```python
from build123d import *

# Parameters (mm, degrees)
BOSS_EXTRUDE1_DEPTH = 1
SKETCH2_R           = 1.6
SKETCH2_W           = 161.4
SKETCH2_H           = 58.6
CUT_EXTRUDE1_DEPTH  = 211.355512163


with BuildPart() as part:
    # Sketch1 → Boss-Extrude1 (new body)
    with BuildSketch(Plane(origin=(0, 0, 0), x_dir=(1, 0, 0), z_dir=(0, 1, 0))):
        with BuildLine():
            Line((92, 0), (-92, 0))
            add(Edge.make_bspline(
                [(-92, 0), (-99, 0), (-100, 8)],
                knots=[0, 0, 0, 1, 1, 1], degree=2))
            add(Edge.make_bspline(
                [(-100, 8), (-109.749547472, 87.403692131), (-94, 164)],
                knots=[0, 0, 0, 1, 1, 1], degree=2))
            add(Edge.make_bspline(
                [(-94, 164), (-90, 183), (-80, 183)],
                knots=[0, 0, 0, 1, 1, 1], degree=2))
            Line((-80, 183), (80, 183))
            add(Edge.make_bspline(
                [(94, 164), (90, 183), (80, 183)],
                knots=[0, 0, 0, 1, 1, 1], degree=2))
            add(Edge.make_bspline(
                [(100, 8), (109.749547472, 87.403692131), (94, 164)],
                knots=[0, 0, 0, 1, 1, 1], degree=2))
            add(Edge.make_bspline(
                [(92, 0), (99, 0), (100, 8)],
                knots=[0, 0, 0, 1, 1, 1], degree=2))
        make_face()
    extrude(amount=BOSS_EXTRUDE1_DEPTH)

    # Sketch2 → Cut-Extrude1 (cut, through all)
    with BuildSketch(Plane(origin=(0, 1, 0), x_dir=(1, 0, 0), z_dir=(0, 1, 0))):
        with Locations(Location((-88, 3.5, 0), (0, 0, 270))):
            Circle(SKETCH2_R)
        with Locations(Location((88, 3.5, 0), (0, 0, 90))):
            Circle(SKETCH2_R)
        with Locations(Location((-80, 175, 0), (0, 0, 270))):
            Circle(SKETCH2_R)
        with Locations(Location((80, 175, 0), (0, 0, 90))):
            Circle(SKETCH2_R)
        with Locations(Location((-88, 68.5, 0), (0, 0, 270))):
            Circle(SKETCH2_R)
        with Locations(Location((88, 68.5, 0), (0, 0, 270))):
            Circle(SKETCH2_R)
        with Locations((-1.3, 43.6)):
            Rectangle(SKETCH2_W, SKETCH2_H)
    extrude(amount=-CUT_EXTRUDE1_DEPTH, mode=Mode.SUBTRACT)


solid = part.part
```
Work out the finished part from the listing and answer in its coordinate system (mm). Round coordinates to 2 decimals unless told otherwise and drop trailing zeros. Loops run counter-clockwise (first coordinate to the right, second up) from the corner with the lowest first, then second, coordinate; pieces in that order, holes last. Notation, with made-up numbers: M -27,70.5 L 13,70.5 A11 cw 13,87.5 Z; hole C -8.75,-10 d2. An arc over 180 degrees is marked long. One line per question, with ' | ' between items.
Q1. Find section A-A, the plane x = 11.5. Give the vertices of the cut face in (y, z).
Conclusion:
outline: M 0,-183 L 1,-183 L 1,-72.9 L 0,-72.9 Z; M 0,-14.3 L 1,-14.3 L 1,0 L 0,0 Z
Q2. Find section B-B, the plane y = 0.75. State how many separate pieces and enclosed holes the cut face has, then the cut area to 3 significant figures.
Conclusion:
separate pieces: 1 | enclosed holes: 7 | area: 27,100 mm2
Q3. This flat-tipped pin is pushed along its axis until it touches: pin 1 Ø3 at (x, z) = (88, -68.5) entering from +Y. Where does it stop, or does it pass through?
Conclusion:
pin 1: passes through
Q4. Consider line 1 along X through (y, z) = (0.5, -68.5); line 2 along Z through (x, y) = (-58, 0.6); line 3 along X through (y, z) = (0.6, -3.5). Determine where each line is inside the solid, lowest interval first. Write a range as from..to.
Conclusion:
line 1: x = -103.73..-89.6, -86.4..-82, 79.4..86.4, 89.6..103.73 | line 2: z = -183..-72.9, -14.3..0 | line 3: x = -98.64..-89.6, -86.4..86.4, 89.6..98.64
